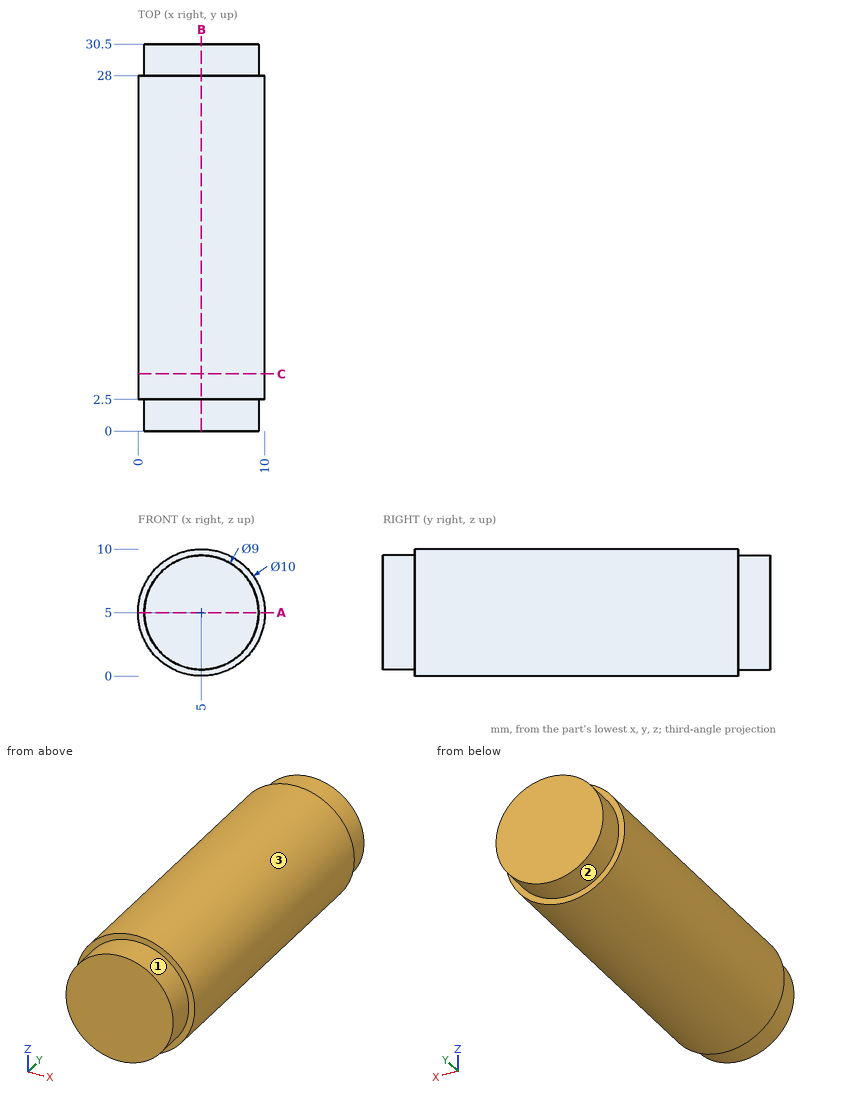
Geometry check sheet. Reference: drawing and pictorial views, mm from the part's lowest x, y, z. A direction names the side the tool comes from. Round coordinates to 2 decimals unless told otherwise and drop trailing zeros. Order: outer loops, then holes, each group sorted by start corner. A loop starts at its lowest first (then second) coordinate and runs counter-clockwise, first axis right, second up. Notation, with made-up numbers: M 55,-5 L 78,-5 A22 cw 78,1 Z; hole C -23.5,-35 d1. An arc over 180 degrees is marked long. Write item = value, one per line.
Q1. Set-up check for the marked faces 1, 2 and 3: record each of +Z, -Z, +X, -X, +Y, -Y from which the full face is reachable in a straight line by a thin tool's end or side.
Answer block:
face_1 = -Y
face_2 = +Y
face_3 = +Y, -Y
Q2. Section check C-C (y = 4.5). Enter the section's corners in (x, z), plus the area to 3 significant figures.
Answer block:
outline = C 5,5 d10
area = 78.5 mm^2
Q3. Scan lines: line 1 (X direction, y = 23, z = 5.25); line 2 (Z direction, x = 6, y = 8.5). Record each from-to range of solid material in increasing order.
Answer block:
line_1 = 0.01 to 9.99
line_2 = 0.1 to 9.9
Q4. Section check B-B (x = 5). Enter the section's corners in (y, z), plus the area to 3 significant figures.
Answer block:
outline = M 0,0.5 L 2.5,0.5 L 2.5,0 L 28,0 L 28,0.5 L 30.5,0.5 L 30.5,9.5 L 28,9.5 L 28,10 L 2.5,10 L 2.5,9.5 L 0,9.5 Z
area = 300 mm^2
Q5. Section check A-A (z = 5). Enter the section's corners in (x, y).
Answer block:
outline = M 0,2.5 L 0.5,2.5 L 0.5,0 L 9.5,0 L 9.5,2.5 L 10,2.5 L 10,28 L 9.5,28 L 9.5,30.5 L 0.5,30.5 L 0.5,28 L 0,28 Z
Q6. Depth check by flat-ended pin: pin 1 Ø4 at (y, z) = (5.5, 1.5) entering from -X; pin 2 Ø2 at (x, z) = (7.5, 1) entering from -Y; pin 3 Ø3 at (x, y) = (9, 23.5) entering from -Z. Enter the tip coordinate at first touch or a pass-through.
Answer block:
pin_1 = 0.23
pin_2 = 0
pin_3 = 0.67
